from build123d import *


with BuildPart() as part:
    # 草图1 → 旋转1 (revolve)
    with BuildSketch(Plane.XY):
        Polygon((0, 8), (8, 8), (8, 1), (3.9, 1), (3.9, 0.4), (2.9, 0.4), (2.9, 5.4), (0, 5.4), align=None)
    revolve(axis=Axis((0, 8, 0), (0, -1, 0)))

    # 草图2 → 切除-旋转1 (revolve, cut)
    with BuildSketch(Plane.XY):
        with BuildLine():
            Line((5, 8), (8, 8))
            Line((8, 8), (8, 7))
            add(Edge.make_bspline(
                [(5, 8), (5.693488859, 8), (7.464893787, 7.980007099), (7.989740211, 7.704714141), (8, 7.515407368), (8, 7)],
                knots=[0, 0, 0, 0, 0.50578806, 0.60578806, 1, 1, 1, 1], degree=3))
        make_face()
    revolve(axis=Axis((0, 0, 0), (0, -1, 0)), mode=Mode.SUBTRACT)


solid = part.part
Geometry: final body of the model. Coordinates: model frame, mm. A direction names the side the tool comes from. Round coordinates to 2 decimals unless told otherwise and drop trailing zeros. Loops run counter-clockwise (first coordinate to the right, second up) from the corner with the lowest first, then second, coordinate; pieces in that order, holes last.
Q1. Pull-direction query (Z, two-part tool) for faces 1 (the flat face through (0, 8, 0)), 2 (the flat face through (0, 5.4, 0)), 3 (the cylindrical face through (-2.87, 0.7, 2.64)); classes: released by +Z, released by -Z, zero draft, split by the parting line, or undercut.
Q2. Section B-B on y = 6.5. Return loops of the section in (x, z), plus the area to 3 significant figures.
Q3. Material intervals for L1, parallel to Z at x = 0, y = 2.85; L2, parallel to Y at x = -1.75, z = -5.25; L3, parallel to X at y = 1.25, z = -1.25, sorted ascending.
Q4. Access query for faces 4 (the flat face through (2, 1, 4)), 5 (the cylindrical face through (-1.73, 3.96, -7.81)). Directions: +Z, -Z, +X, -X, +Y, -Y. A direction counts if a zero-diameter tool reaches every point of the face in a straight line with its end or side. Return the directions, or none.
Q5. Pin query (flat end, axial travel): P1, Ø1, axis at x = 1, z = -0.5, coming from the -Y side; P2, Ø1.5, axis at x = 5, y = 3, coming from the -Z side; P3, Ø1, axis at y = 6.5, z = -2.5, coming from the +X side. Return the tip coordinate at first contact, or that it passes through.
Q6. Section A-A on y = 3.5. Return loops of the section in (x, z), plus the area to 3 significant figures.
Evaluation:
1. face 1: zero draft
1. face 2: undercut
1. face 3: split by the parting line
2. outline: circle Ø16 at (0, 0)
2. area: 201 mm2
3. L1: z = -8 to -2.9, 2.9 to 8
3. L2: y = 1 to 8
3. L3: x = -7.9 to -2.62, 2.62 to 7.9
4. face 4: -Y
4. face 5: +Y, -Y
5. P1: stops at y = 5.4
5. P2: stops at z = -6.78
5. P3: stops at x = 7.75
6. outline: circle Ø16 at (0, 0); hole circle Ø5.8 at (0, 0)
6. area: 175 mm2
